Geometry: final body of the model. Coordinates: model frame, mm. Face numbers are marked on the shaded views. A direction names the side the tool comes from. Give positions to 0.01 mm unless a question says otherwise; leave off trailing zeros. Write each loop counter-clockwise with the first axis right and the second up, starting at its lowest first coordinate (ties: lowest second). Pieces come first, ordered by that corner, then holes.
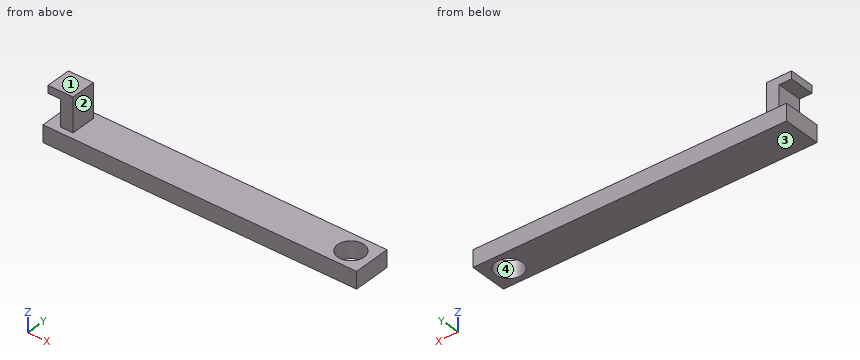
from build123d import *

# Parameters (mm, degrees)
F0_W     = 92.7622355521
F0_H     = 11.1067872494
F0_R     = 3.9563607237
F0_W_2   = 3.7022642791
F0_H_2   = 7.4045229703
F1_DEPTH = 5
F2_DEPTH = 15.1
F3_W     = 7.4045229703
F3_H     = 2.2449219063
F4_DEPTH = 3.7022568285


with BuildPart() as f1:
    # F0 (on Top) → F1 (new body)
    with BuildSketch(Plane.XY):
        with Locations((-1.0284055024, 24.7845901176)):
            Rectangle(F0_W, F0_H)
        Polygon((-40.0050021708, 28.4868516028), (-36.3027378917, 28.4868516028), (-36.3027378917, 21.0823286325), (-40.0050021708, 21.0823286325), (-43.7072664499, 21.0823286325), (-43.7072664499, 28.4868516028), align=None, mode=Mode.SUBTRACT)
        with Locations((39.1822755337, 24.7845901176)):
            Circle(F0_R, mode=Mode.SUBTRACT)
        with Locations((-38.1538700312, 24.7845901176)):
            Rectangle(F0_W_2, F0_H_2)
    extrude(amount=F1_DEPTH)

    # F0 (on Top) → F2 (join)
    with BuildSketch(Plane.XY):
        with Locations((-41.8561343104, 24.7845901176)):
            Rectangle(F0_W_2, F0_H_2)
    extrude(amount=F2_DEPTH)

    # F3 (on face) → F4 (join, through all)
    with BuildSketch(Plane(origin=(-43.7072664499, 0, 0), x_dir=(0, -1, 0), z_dir=(-1, 0, 0))):
        with Locations((-24.7845901176, 13.9775390469)):
            Rectangle(F3_W, F3_H)
    extrude(amount=F4_DEPTH)


solid = f1.part
Q1. Section D-D on z = 9.25. Output: boundary loops of the cut face in (x, y) (3 decimals), plus the area to 3 significant figures.
Filled sheet:
outline: (-43.707, 21.082) - (-40.005, 21.082) - (-40.005, 28.487) - (-43.707, 28.487) - close
area: 27.4 mm2
Q2. Section C-C on x = 39. Output: boundary loops of the cut face in (y, z), plus the area to 3 significant figures.
Filled sheet:
outline: (19.23, 0) - (20.83, 0) - (20.83, 5) - (19.23, 5) - close; (28.74, 0) - (30.34, 0) - (30.34, 5) - (28.74, 5) - close
area: 16.0 mm2
Q3. Ray query, line 1 along Z through (x, y) = (-13, 25.5); line 2 along Y through (x, z) = (-41, 8); line 3 along X through (y, z) = (22, 12) (3 decimals). Return the intervals inside material, ascending.
Filled sheet:
line 1: z = 0 to 5
line 2: y = 21.08 to 28.49
line 3: x = -43.707 to -40.005
Q4. Section A-A on y = 26.25. Output: boundary loops of the cut face in (x, z) (3 decimals).
Filled sheet:
outline: (-47.41, 0) - (35.507, 0) - (35.507, 5) - (-40.005, 5) - (-40.005, 15.1) - (-47.41, 15.1) - (-47.41, 12.855) - (-43.707, 12.855) - (-43.707, 5) - (-47.41, 5) - close; (42.857, 0) - (45.353, 0) - (45.353, 5) - (42.857, 5) - close
Q5. Access query for the marked faces 1 and 2. Directions: +Z, -Z, +X, -X, +Y, -Y. A direction counts if a zero-diameter tool reaches every point of the face in a straight line with its end or side. Return the directions, or none.
Filled sheet:
face 1: +Z, +X, -X, +Y, -Y
face 2: +Z, +X, +Y, -Y
Q6. Pin query (flat end, axial travel): P1, Ø3.5, axis at x = -4, y = 23.5, coming from the +Z side; P2, Ø6, axis at y = 25.5, z = 9, coming from the -X side; P3, Ø8, axis at x = -42, z = 10.5, coming from the -Y side. Return the tip coordinate at first contact, or that it passes through.
Filled sheet:
P1: stops at z = 5
P2: stops at x = -43.71
P3: stops at y = 21.08
Q7. Pull-direction query (Y, two-part tool) for the marked faces 3 and 4; classes: released by +Y, released by -Y, zero draft, split by the parting line, or undercut.
Filled sheet:
face 3: zero draft
face 4: undercut
Q8. Section B-B on z = 2.5. Output: boundary loops of the cut face in (x, y), plus the area to 3 significant figures.
Filled sheet:
outline: (-47.41, 19.23) - (45.35, 19.23) - (45.35, 30.34) - (-47.41, 30.34) - close; hole circle Ø7.91 at (39.18, 24.78)
area: 981 mm2
